Input: dimensioned drawing with shaded views. Units: mm. Origin: part minimum x, y, z. Round coordinates to 2 decimals unless told otherwise and drop trailing zeros. Order: outer loops, then holes, each group sorted by start corner. A loop starts at its lowest first (then second) coordinate and runs counter-clockwise, first axis right, second up. Notation, with made-up numbers: (81, -31.75) - (140, -31.75) arc R27 cw to (140, 7.25) - close; hole circle Ø8 at (26, 65). An arc over 180 degrees is marked (long way). Put each result on its own line as item: value. Start each with the question number.
(1) Material intervals for L1, parallel to X at y = 7.25, z = 0.6; L2, parallel to Y at x = 36.22, z = 1.1; L3, parallel to X at y = 5.25, z = 0.1, sorted ascending. Write a range as [from, to].
(2) Section D-D (x = 36.22). Output: boundary loops of the cut face in (y, z).
(3) Pin query (flat end, axial travel): P1, Ø6.5, axis at x = 69.5, y = 7.5, coming from the -Z side. Return the tip coordinate at first contact, or that it passes through.
(4) Section B-B (y = 7.5). Output: boundary loops of the cut face in (x, z), and give its area (3 significant figures).
(5) Section C-C (z = 0.6). Output: boundary loops of the cut face in (x, y), and give its area (3 significant figures).
(6) Section A-A (x = 5.5). Output: boundary loops of the cut face in (y, z).
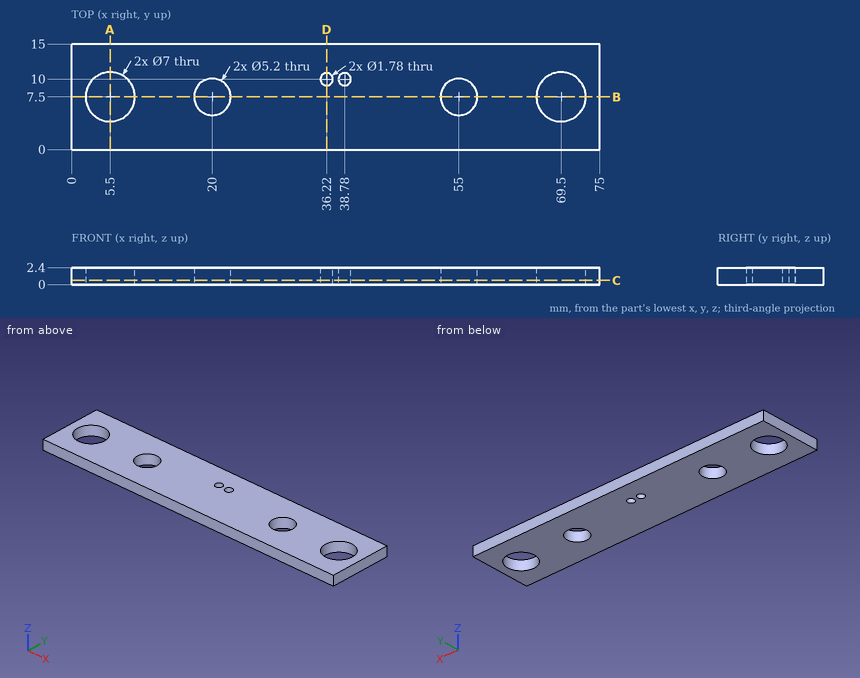
Checks:
1. L1: x = [0, 2.01], [8.99, 17.41], [22.59, 52.41], [57.59, 66.01], [72.99, 75]
1. L2: y = [0, 9.11], [10.89, 15]
1. L3: x = [0, 2.82], [8.18, 18.7], [21.3, 53.7], [56.3, 66.82], [72.18, 75]
2. outline: (0, 0) - (9.11, 0) - (9.11, 2.4) - (0, 2.4) - close; (10.89, 0) - (15, 0) - (15, 2.4) - (10.89, 2.4) - close
3. P1: passes through
4. outline: (0, 0) - (2, 0) - (2, 2.4) - (0, 2.4) - close; (9, 0) - (17.4, 0) - (17.4, 2.4) - (9, 2.4) - close; (22.6, 0) - (52.4, 0) - (52.4, 2.4) - (22.6, 2.4) - close; (57.6, 0) - (66, 0) - (66, 2.4) - (57.6, 2.4) - close; (73, 0) - (75, 0) - (75, 2.4) - (73, 2.4) - close
4. area: 121 mm²
5. outline: (0, 0) - (75, 0) - (75, 15) - (0, 15) - close; hole circle Ø7 at (5.5, 7.5); hole circle Ø5.2 at (20, 7.5); hole circle Ø1.78 at (36.22, 10); hole circle Ø1.78 at (38.78, 10); hole circle Ø5.2 at (55, 7.5); hole circle Ø7 at (69.5, 7.5)
5. area: 1,000 mm²
6. outline: (0, 0) - (4, 0) - (4, 2.4) - (0, 2.4) - close; (11, 0) - (15, 0) - (15, 2.4) - (11, 2.4) - close
